```python
from build123d import *

# Parameters (mm, degrees)
ESBO_O1_R                = 5.857023813
RESSALTO_EXTRUS_O1_DEPTH = 2


with BuildPart() as part:
    # Esboço1 → Ressalto-extrusão1 (new body)
    with BuildSketch(Plane(origin=(0, 0, 0), x_dir=(1, 0, 0), z_dir=(0, 1, 0))):
        Polygon((-20, 48), (-39, 30), (-39, -30), (39, -30), (39, 30), (20, 48), (20, 28), (-20, 28), align=None)
        with Locations(Location((-20, -15.384615385, 0), (0, 0, 270))):
            Circle(ESBO_O1_R, mode=Mode.SUBTRACT)
        with Locations(Location((20, -15.384615385, 0), (0, 0, 90))):
            Circle(ESBO_O1_R, mode=Mode.SUBTRACT)
    extrude(amount=RESSALTO_EXTRUS_O1_DEPTH)


solid = part.part
```
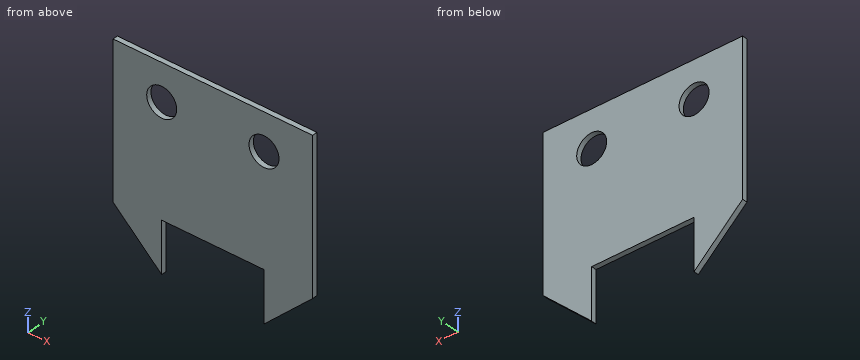
Input: part model. Units: mm. Frame: model coordinates. Round coordinates to 2 decimals unless told otherwise and drop trailing zeros. Loops run counter-clockwise (first coordinate to the right, second up) from the corner with the lowest first, then second, coordinate; pieces in that order, holes last. Notation, with made-up numbers: (41, 60.25) -> (94, 60.25) arc R24 ccw to (94, 91.25) -> close; hole circle Ø7 at (15, 11). An arc over 180 degrees is marked (long way). Use one line per item in the form item = value. Start each with the question number.
Item 1: Section query C-C on z = 18. Return the cut outline in (x, y).
Item 2: Section query B-B on y = 0.95. Return the cut outline in (x, z).
Item 3: Material intervals for L1, parallel to X at y = 1.95, z = -30; L2, parallel to Z at x = -8.5, y = 1.3; L3, parallel to X at y = 0.8, z = 13, sorted ascending. Write a range as from..to.
Item 4: Section query D-D on x = -10.5. Return the cut outline in (y, z).
Item 5: Contact query for a flat-ended pin moving along its axis: pin 1 Ø9.5 at (x, z) = (-20, 15.38) entering from +Y. Output: stop coordinate, or through.
Item 6: Section query A-A on x = 16. Return the cut outline in (y, z).
Ans:
q1.outline = (-39, 0) -> (-25.24, 0) -> (-25.24, 2) -> (-39, 2) -> close; (-14.76, 0) -> (14.76, 0) -> (14.76, 2) -> (-14.76, 2) -> close; (25.24, 0) -> (39, 0) -> (39, 2) -> (25.24, 2) -> close
q2.outline = (-39, -30) -> (-20, -48) -> (-20, -28) -> (20, -28) -> (20, -48) -> (39, -30) -> (39, 30) -> (-39, 30) -> close; hole circle Ø11.71 at (-20, 15.38); hole circle Ø11.71 at (20, 15.38)
q3.L1 = -39..-20, 20..39
q3.L2 = -28..30
q3.L3 = -39..-25.35, -14.65..14.65, 25.35..39
q4.outline = (0, -28) -> (2, -28) -> (2, 30) -> (0, 30) -> close
q5.pin_1 = through
q6.outline = (0, -28) -> (2, -28) -> (2, 11.11) -> (0, 11.11) -> close; (0, 19.66) -> (2, 19.66) -> (2, 30) -> (0, 30) -> close
